Design review of the part shown in the three views and the two pictorial views. Dimensions are in mm from the part's minimum x, y and z. Round coordinates to 2 decimals unless told otherwise and drop trailing zeros. Loops run counter-clockwise (first coordinate to the right, second up) from the corner with the lowest first, then second, coordinate; pieces in that order, holes last.
1. Consider section C-C on y = 25. State the section outline as (x, z) points, then the cut area to 3 significant figures.
2. To check wall thickness, follow line 1 along Y through (x, z) = (123.5, 35); line 2 along Z through (x, y) = (25, 18.5); line 3 along Z through (x, y) = (115.5, 27.5). State the ranges of each line that lie inside material, in increasing order.
3. Consider section A-A on z = 35. State the section outline as (x, y) points, then the cut area to 3 significant figures.
4. Consider section B-B on x = 36. State the section outline as (y, z) points.
5. Clearance check with a flat-ended pin moving along its axis: pin 1 Ø17.5 at (y, z) = (25, 35) entering from -X. State where the tip first meets the part, or that it passes through.
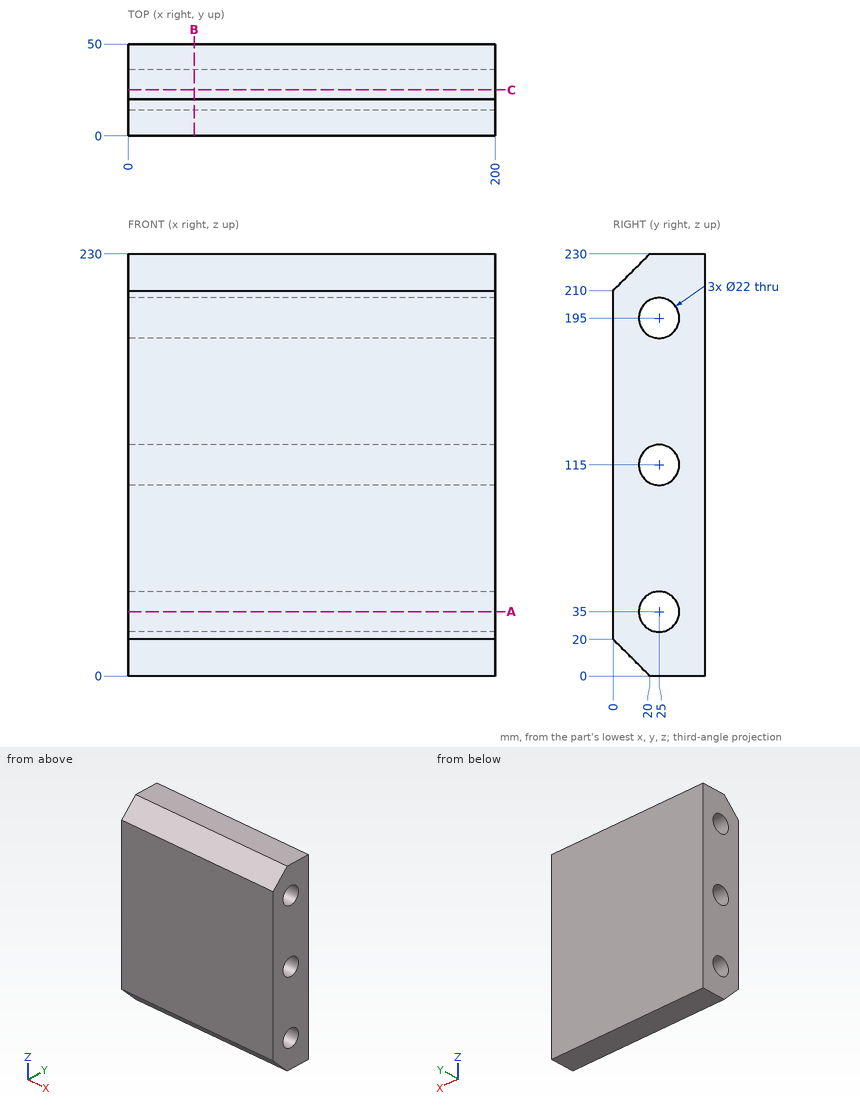
Resolved:
1. outline: (0, 0) - (200, 0) - (200, 24) - (0, 24) - close; (0, 46) - (200, 46) - (200, 104) - (0, 104) - close; (0, 126) - (200, 126) - (200, 184) - (0, 184) - close; (0, 206) - (200, 206) - (200, 230) - (0, 230) - close
1. area: 32,800 mm2
2. line 1: y = 0 to 14, 36 to 50
2. line 2: z = 1.5 to 26.13, 43.87 to 106.13, 123.87 to 186.13, 203.87 to 228.5
2. line 3: z = 0 to 24.29, 45.71 to 104.29, 125.71 to 184.29, 205.71 to 230
3. outline: (0, 0) - (200, 0) - (200, 14) - (0, 14) - close; (0, 36) - (200, 36) - (200, 50) - (0, 50) - close
3. area: 5,600 mm2
4. outline: (0, 20) - (20, 0) - (50, 0) - (50, 230) - (20, 230) - (0, 210) - close; hole circle Ø22 at (25, 35); hole circle Ø22 at (25, 115); hole circle Ø22 at (25, 195)
5. pin 1: passes through
